Geometry check sheet. Reference: the model listing, model coordinates, mm. Face numbers are marked on the shaded views. A direction names the side the tool comes from. Round coordinates to 2 decimals unless told otherwise and drop trailing zeros. Loops run counter-clockwise (first coordinate to the right, second up) from the corner with the lowest first, then second, coordinate; pieces in that order, holes last. Notation, with made-up numbers: (24.25, 55.5) -> (29.25, 55.5) arc R16 ccw to (29.25, 80.5) -> close; hole circle Ø6 at (15, 54). An arc over 180 degrees is marked (long way). Use a Markdown table: item, result. Add a question column.
Q1. Sectioned sample at A-A, the plane z = 6.5. Give the number of separate pieces and of enclosed holes in the cut face, then the cut area to 3 significant figures.
Q2. Set-up check for the marked faces 1, 2, 3 and 4: record each of +Z, -Z, +X, -X, +Y, -Y from which the full face is reachable in a straight line by a thin tool's end or side.
Q3. Sectioned sample at B-B, the plane x = 8. Enter the section's corners in (y, z).
Q4. Sectioned sample at D-D, the plane y = -0.5. Enter the section's corners in (x, z), then the cut area to 3 significant figures.
Q5. Gauge pin test, flat ends, axial feed: P1, Ø9.5, axis at x = -11.09, y = 19.12, coming from the +Z side; P2, Ø1.5, axis at y = -3, z = 5.5, coming from the -X side; P3, Ø4, axis at x = -24, y = -8.5, coming from the -Z side; P4, Ø5, axis at y = 0, z = 3, coming from the +X side. Record the tip position at first contact, or that the pin passes through.
Q6. Sectioned sample at C-C, the plane z = 1.5. Enter the section's corners in (x, y).
Q7. Material ranges on L1, parallel to Y at x = -2.5, z = 4.25; L2, parallel to Y at x = -11, z = 8.5; L3, parallel to Y at x = 11, z = 7.25, recorded low to high.
Q8. Release check for a two-part mould opening along X. For the marked faces 5, 6, 7 and 8 record: released by +X, released by -X, zero draft, split by the parting line, or undercut.
```python
from build123d import *

# Parameters (mm, degrees)
F1_DEPTH = 13
F2_R     = 1.5
F3_DEPTH = 12.5
F4_R     = 2.2
F5_DEPTH = 8
F7_R     = 1.75
F6_R     = 1.75
F8_DEPTH = 25
F9_R     = 3


with BuildPart() as f1:
    # F0 (on Top) → F1 (new body)
    with BuildSketch(Plane.XY):
        with BuildLine():
            Line((-31.585052, -11.882249), (-31.585052, -17.882249))
            Line((-31.585052, -17.882249), (13.414948, -17.882249))
            Line((13.414948, -17.882249), (13.414948, -11.882249))
            Line((13.414948, -11.882249), (0.914948, -11.882249))
            Line((0.914948, -11.882249), (0.914948, 18.208811))
            Line((0.914948, 18.208811), (-7.035814, 18.208811))
            ThreePointArc((-7.035814, 18.208811), (-15.235052, 19.117751), (-7.035814, 20.02669))
            Line((-7.035814, 20.02669), (0.914948, 20.02669))
            Line((0.914948, 20.02669), (0.914948, 27.117751))
            Line((0.914948, 27.117751), (-11.085052, 27.117751))
            ThreePointArc((-11.085052, 27.117751), (-16.741906, 24.774605), (-19.085052, 19.117751))
            Line((-19.085052, 19.117751), (-19.085052, -11.882249))
            Line((-19.085052, -11.882249), (-31.585052, -11.882249))
        make_face()
    extrude(amount=F1_DEPTH)

    # F2 (on face) → F3 (cut, symmetric)
    with BuildSketch(Plane(origin=(0, 18.208811, 0), x_dir=(-1, 0, 0), z_dir=(0, 1, 0))):
        with Locations((3.060433, 6.5)):
            Circle(F2_R)
    extrude(amount=F3_DEPTH, both=True, mode=Mode.SUBTRACT)

    # F4 (on face) → F5 (cut)
    with BuildSketch(Plane(origin=(0, 27.117751, 0), x_dir=(-1, 0, 0), z_dir=(0, 1, 0))):
        with Locations((3.060433, 6.5)):
            Circle(F4_R)
    extrude(amount=-F5_DEPTH, mode=Mode.SUBTRACT)

    # F7 (on face) + F6 (on face) → F8 (cut)
    with BuildSketch(Plane(origin=(0, -11.882249, 0), x_dir=(-1, 0, 0), z_dir=(0, 1, 0))):
        with Locations((25.335052, 6.5)):
            Circle(F7_R)
    with BuildSketch(Plane(origin=(0, -11.882249, 0), x_dir=(-1, 0, 0), z_dir=(0, 1, 0))):
        with Locations((-7.164948, 6.5)):
            Circle(F6_R)
    extrude(amount=-F8_DEPTH, mode=Mode.SUBTRACT)

    # F9
    f9_edges = [f1.edges().sort_by_distance(p)[0] for p in [
        (13.414948, -14.882249, 13),
        (-31.585052, -14.882249, 13),
        (0.914948, 3.163281, 13),
        (0.914948, 23.57222, 13),
        (-19.085052, 3.617751, 13),
    ]]
    fillet(f9_edges, radius=F9_R)


solid = f1.part
```
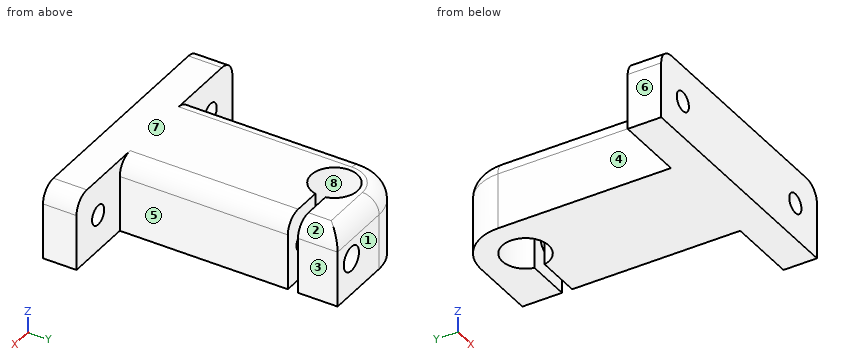
Values:
| question | item | result |
|---|---|---|
| 1 | separate pieces | 4 |
| 1 | enclosed holes | 0 |
| 1 | area | 857 mm^2 |
| 2 | face 1 | +Z, -Z, +X, -X, +Y |
| 2 | face 2 | +Z, +X, +Y |
| 2 | face 3 | +Z, -Z, +X, +Y |
| 2 | face 4 | +Z, -Z, -X, +Y |
| 3 | outline | (-17.88, 0) -> (-11.88, 0) -> (-11.88, 4.96) -> (-17.88, 4.96) -> close; (-17.88, 8.04) -> (-11.88, 8.04) -> (-11.88, 13) -> (-17.88, 13) -> close |
| 4 | outline | (-19.09, 0) -> (0.91, 0) -> (0.91, 10) arc R3 ccw to (-2.09, 13) -> (-16.09, 13) arc R3 ccw to (-19.09, 10) -> close |
| 4 | area | 256 mm^2 |
| 5 | P1 | z = 13 |
| 5 | P2 | x = -19.09 |
| 5 | P3 | through |
| 5 | P4 | x = 0.91 |
| 6 | outline | (-31.59, -17.88) -> (13.41, -17.88) -> (13.41, -11.88) -> (0.91, -11.88) -> (0.91, 18.21) -> (-7.04, 18.21) arc R4.15 cw (long way) to (-7.04, 20.03) -> (0.91, 20.03) -> (0.91, 27.12) -> (-11.09, 27.12) arc R8 ccw to (-19.09, 19.12) -> (-19.09, -11.88) -> (-31.59, -11.88) -> close |
| 7 | L1 | -17.88 to 18.21, 20.03 to 27.12 |
| 7 | L2 | -17.88 to 14.97, 23.27 to 27.12 |
| 7 | L3 | -17.88 to -11.88 |
| 8 | face 5 | released by +X |
| 8 | face 6 | released by -X |
| 8 | face 7 | zero draft |
| 8 | face 8 | undercut |
